Autodesk Fusion 360 part; units mm, degrees
sketch "Sketch1" plane through (0, 0, 0) normal (0, 0, 1) x (1, 0, 0)
  line L0 (10, 0) -> (30, 0)
  line L1 (40, 10) -> (40, 30)
  line L2 (30, 40) -> (10, 40)
  line L3 (0, 30) -> (0, 10)
  line L4 (10, -5) -> (30, -5)
  line L5 (45, 10) -> (45, 30)
  line L6 (30, 45) -> (10, 45)
  line L7 (-5, 30) -> (-5, 10)
  arc A0 (10, 40) -> (0, 30) centre (10, 30) ccw
  arc A1 (40, 30) -> (30, 40) centre (30, 30) ccw
  arc A2 (30, 0) -> (40, 10) centre (30, 10) ccw
  arc A3 (0, 10) -> (10, 0) centre (10, 10) ccw
  arc A4 (45, 30) -> (30, 45) centre (30, 30) ccw
  arc A5 (30, -5) -> (45, 10) centre (30, 10) ccw
  arc A6 (-5, 10) -> (10, -5) centre (10, 10) ccw
  arc A7 (10, 45) -> (-5, 30) centre (10, 30) ccw
  circle A8 centre (20, 0) radius 1
  circle A9 centre (40, 20) radius 1
  circle A10 centre (20, 40) radius 1
  circle A11 centre (0, 20) radius 1
  point P0 (40, 0)
  point P1 (0, 40)
  dimension "d1" = 40
  dimension "d2" = 40
  dimension "d3" = 10
  dimension "d4" = 15
extrude "Extrude1" add sketch "Sketch1" along normal blind 10 contours L0 L1 L2 L3 A0 A1 A2 A3 A8 A9 A10 A11 | L0 A8 | L0 A8 | L1 A9 | L1 A9 | L3 A11 | L3 A11 | L2 A10 | L2 A10
extrude "Extrude2" add sketch "Sketch1" along normal blind 5 contours L0 A8 | L1 A9 | L3 A11 | L2 A10 | L4 L5 L6 L7 A4 A5 A6 A7 picked at (19.774, -0.5035) picked at (40.3032, 20.1385) picked at (-0.4549, 20.2371) picked at (20.2754, 40.3843)
Read the model definition and answer for the solid it produces. Units are mm, in the model's axes. A direction names the side the tool comes from. Round coordinates to 2 decimals unless told otherwise and drop trailing zeros. Write each loop counter-clockwise with the first axis right and the second up, starting at its lowest first coordinate (ties: lowest second). Pieces come first, ordered by that corner, then holes.
1. The part is cut by section B-B, the plane x = 16. Determine the outline of the cut face in (y, z), then the cut area to 3 significant figures.
2. The part is cut by section C-C, the plane z = 7.25. Determine the outline of the cut face in (x, y), then the cut area to 3 significant figures.
3. The part is cut by section A-A, the plane y = 20. Determine the outline of the cut face in (x, z).
4. Which of the six approach directions +Z, -Z, +X, -X, +Y, -Y give full straight-line access (tool end or side, diameter ignored) to faces 1 (the face through (2.85, 36.99, 7.46)), 2 (the face through (20, -1, 7)), 3 (the face through (21.7, 40.5, 5)), 4 (the face through (-1, 20, 7)), 5 (the face through (41, 20, 7))?
5. Straight lines are drawn through the part: L1, parallel to Y at x = 9.5, z = 5.75; L2, parallel to X at y = 28.5, z = 7.25; L3, parallel to Z at x = 0.5, y = 34. For each, find the intervals that lie inside material, in ascending order.
6. Given pin 1 Ø5.5 at (y, z) = (25, 8) entering from -X; pin 2 Ø1 at (x, z) = (34.5, 3.5) entering from +Y; pin 3 Ø5 at (x, z) = (1.5, 9) entering from +Y, each flat-ended and moving along its own axis, determine where each tip first touches the part or whether it passes through.
Values:
1. outline: (-5, 0) - (45, 0) - (45, 5) - (40, 5) - (40, 10) - (0, 10) - (0, 5) - (-5, 5) - close
1. area: 450 mm2
2. outline: (0, 10) arc R10 ccw to (10, 0) - (19, 0) arc R1 ccw to (21, 0) - (30, 0) arc R10 ccw to (40, 10) - (40, 19) arc R1 ccw to (40, 21) - (40, 30) arc R10 ccw to (30, 40) - (21, 40) arc R1 ccw to (19, 40) - (10, 40) arc R10 ccw to (0, 30) - (0, 21) arc R1 ccw to (0, 19) - close
2. area: 1,520 mm2
3. outline: (-5, 0) - (45, 0) - (45, 5) - (41, 5) - (41, 10) - (-1, 10) - (-1, 5) - (-5, 5) - close
4. face 1: +Z, -X, +Y
4. face 2: +Z, -Y
4. face 3: +Z
4. face 4: +Z, -X
4. face 5: +Z, +X
5. L1: y = 0.01 to 39.99
5. L2: x = 0 to 40
5. L3: z = 0 to 5
6. pin 1: stops at x = 0
6. pin 2: stops at y = 44.46
6. pin 3: stops at y = 38
